Autodesk Inventor part; units mm, degrees
ref_plane "YZ Plane" through (0, 0, 0) normal (1, 0, 0) x (0, 1, 0)
ref_plane "XZ Plane" through (0, 0, 0) normal (0, 1, 0) x (-1, 0, 0)
ref_plane "XY Plane" through (0, 0, 0) normal (0, 0, 1) x (1, 0, 0)
sketch "Sketch1" plane through (0, 0, 0) normal (0, 1, 0) x (-1, 0, 0)
  point P0 (0, 0)
sketch "Sketch2" plane through (0, 0, 0) normal (0, 1, 0) x (-1, 0, 0)
  line L0 (0, 0) -> (16, 0)
  line L1 (16, 0) -> (16, -16)
  line L2 (16, -16) -> (0, -16)
  line L3 (0, -16) -> (0, 0)
  line L4 (0, 0) -> (0, -8)
  dimension "d1" = 16
  dimension "d2" = 16
extrude "Extrusion1" add sketch "Sketch2" along normal blind 16
ref_plane "Work Plane1" through (-8, 0, 0) normal (1, 0, 0) x (0, 0, -1)
sketch "Sketch5" plane through (-8, 0, 0) normal (1, 0, 0) x (0, 0, -1)
  line L0 (0, 0) -> (16, 0)
  line L1 (11.3, 0) -> (4.7, 0)
  line L2 (8, 0) -> (11.3, 0)
  line L3 (11.3, 0) -> (11.3, 3.4)
  line L4 (11.3, 3.4) -> (10.9, 3.4)
  line L5 (11.3, 0) -> (11.3, 3.3)
  line L6 (10.9, 3.4) -> (11.3, 0)
  line L7 (11.3, 3.3) -> (8, 6.6)
  line L8 (8, 0) -> (8, 6.6)
  line L9 (10.9, 3.4) -> (8, 6.3)
  line L10 (16, 0) -> (0, 0)
  line L11 (5.1, 3.4) -> (4.7, 0)
  line L12 (5.1, 3.4) -> (8, 6.3)
  dimension "d39" = 3.3
  dimension "d40" = 3.4
  dimension "d41" = 0.4
  dimension "d42" = 6.6
extrude "Extrusion4" cut sketch "Sketch5" along normal mid plane 13 contours L11 L12 L8 L0 | L8 L9 L6 L0
properties part number "pawn"
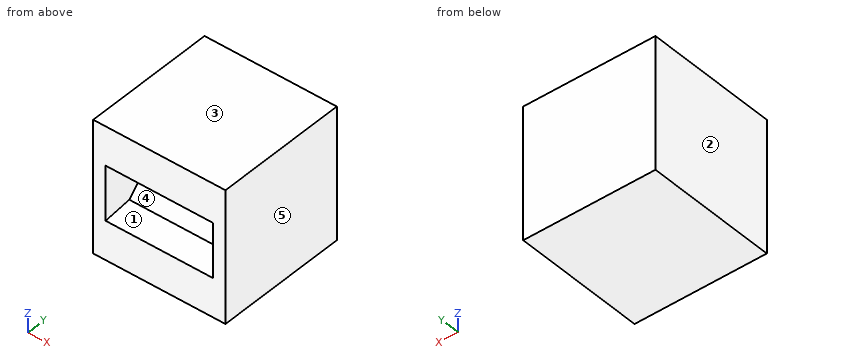
Verification items for the finished model (mm, model axes). Face numbers are marked on the shaded views. A direction names the side the tool comes from. Give positions to 0.01 mm unless a question says otherwise; leave off trailing zeros. Loops run counter-clockwise (first coordinate to the right, second up) from the corner with the lowest first, then second, coordinate; pieces in that order, holes last. Notation, with made-up numbers: (4, 22.5) - (47, 22.5) arc R18 cw to (47, 45.5) - close; hole circle Ø1 at (32.5, -7). An arc over 180 degrees is marked (long way). Write each question's results on one line, items separated by ' | '.
1) Depth check by flat-ended pin: P1, Ø4, axis at x = -8, z = -10, coming from the -Y side. Enter the tip coordinate at first touch or a pass-through.
Solution:
P1: y = 0
2) Sectioned sample at A-A on y = 6. Record the boundary of the cut face in (x, z).
Solution:
outline: (-16, -16) - (0, -16) - (0, 0) - (-16, 0) - close; hole (-14.5, -8.3) - (-1.5, -8.3) - (-1.5, -7.7) - (-14.5, -7.7) - close
3) Tool access check on the marked faces 1 and 2. Record the directions out of +Z, -Z, +X, -X, +Y, -Y that give a thin tool (end or side, any length) a straight path to the whole face; none if there is none.
Solution:
face 1: -Y | face 2: +Z, -Z, -X, +Y, -Y
4) Sectioned sample at D-D on y = 4. Record the boundary of the cut face in (x, z), plus the area to 3 significant figures.
Solution:
outline: (-16, -16) - (0, -16) - (0, 0) - (-16, 0) - close; hole (-14.5, -10.3) - (-1.5, -10.3) - (-1.5, -5.7) - (-14.5, -5.7) - close | area: 196 mm2
5) Sectioned sample at B-B on z = -9.75. Record the boundary of the cut face in (x, y), plus the area to 3 significant figures.
Solution:
outline: (-16, 0) - (-14.5, 0) - (-14.5, 4.55) - (-1.5, 4.55) - (-1.5, 0) - (0, 0) - (0, 16) - (-16, 16) - close | area: 197 mm2
6) Material ranges on L1, parallel to X at y = 3.5, z = -7.75; L2, parallel to Z at x = -13.5, y = 3; L3, parallel to Z at x = -2.25, y = 4.25, recorded low to high. Write a range as from..to.
Solution:
L1: -16..-14.5, -1.5..0 | L2: -16..-10.95, -5.05..0 | L3: -16..-10.05, -5.95..0
7) Sectioned sample at C-C on x = -1.75. Record the boundary of the cut face in (y, z).
Solution:
outline: (0, -16) - (16, -16) - (16, 0) - (0, 0) - (0, -4.7) - (3.4, -5.1) - (6.3, -8) - (3.4, -10.9) - (0, -11.3) - close
8) Mould release check, pull along Z, two halves, no side actions. Record for the marked faces 3, 4 and 5: pulls with the +Z half, pulls with the -Z half, needs draft (parallel to the pull), parting line crosses it, or undercut.
Solution:
face 3: pulls with the +Z half | face 4: undercut | face 5: needs draft
